The model under review builds one solid part; all positions refer to its coordinate system, in mm. Face numbers are marked on the shaded views. A direction names the side the tool comes from. Round coordinates to 2 decimals unless told otherwise and drop trailing zeros. Loops run counter-clockwise (first coordinate to the right, second up) from the corner with the lowest first, then second, coordinate; pieces in that order, holes last. Notation, with made-up numbers: M -30.75,21.5 L 7.25,21.5 A7 ccw 7.25,27.5 Z; hole C 62,63.5 d5. An arc over 180 degrees is marked long. Use a Markdown table: item, result. Add a question column.
```python
from build123d import *

# Parameters (mm, degrees)
SKETCH1_R                = 5.875
BASE_FLANGE2_DEPTH       = 2.85
TAB1_START               = -2.85
TAB1_DEPTH               = 2.85
FILLET1_R                = 0.5
CIRPATTERN1_COUNT        = 10
FILLET1_OF_CIRPATTERN1_R = 0.5
CUT_EXTRUDE1_DEPTH       = 13.516657182


# Read off the part's stored shape, not the designer's step: Tab1
# Sheet-metal steps are written as plain solids
with BuildPart() as part:
    # Sketch1 → Base-Flange2 (new body)
    with BuildSketch(Plane(origin=(0, 0, 0), x_dir=(1, 0, 0), z_dir=(0, 1, 0))):
        with Locations(Location((0, 0, 0), (0, 0, 270))):
            Circle(SKETCH1_R)
    extrude(amount=-BASE_FLANGE2_DEPTH)

    # Tab1 outline → Tab1 (add)
    with BuildSketch(Plane(origin=(0, 0, 0), x_dir=(1, 0, 0), z_dir=(0, 1, 0)).offset(TAB1_START)):
        with BuildLine():
            ThreePointArc((0.4, 8.79090439), (0, 8.8), (-0.4, 8.79090439))
            ThreePointArc((-0.4, 8.79090439), (-1.1629301, 7.310892011), (-1.5, 5.680283884))
            ThreePointArc((-1.5, 5.680283884), (0, 5.875), (1.5, 5.680283884))
            ThreePointArc((1.5, 5.680283884), (1.1629301, 7.310892011), (0.4, 8.79090439))
        make_face()
    tab1 = extrude(amount=TAB1_DEPTH)

    # Fillet1
    fillet1_edges = [part.edges().sort_by_distance(p)[0] for p in [
        (-1.5, -1.425, -5.680283884),
        (-0.4, -1.425, -8.79090439),
        (0.4, -1.425, -8.79090439),
        (1.5, -1.425, -5.680283884),
    ]]
    fillet(fillet1_edges, radius=FILLET1_R)

    # CirPattern1: Tab1 ×10 about axis
    cirpattern1_axis = Axis((0, 0, 0), (0, 1, 0))
    for i in range(1, CIRPATTERN1_COUNT):
        add(tab1.rotate(cirpattern1_axis, i * 360 / CIRPATTERN1_COUNT))

    # Fillet1 of CirPattern1
    fillet1_of_cirpattern1_edges = [part.edges().sort_by_distance(p)[0] for p in [
        (-4.552312587, -1.425, -3.713768317),
        (-5.490770753, -1.425, -6.876876947),
        (-4.843557157, -1.425, -7.347105148),
        (-2.125261604, -1.425, -5.477124073),
        (-5.865796494, -1.425, -0.328719479),
        (-8.484253702, -1.425, -2.336116246),
        (-8.237040106, -1.425, -3.096961459),
        (-4.938745511, -1.425, -3.181889027),
        (-4.938745511, -1.425, 3.181889027),
        (-8.237040106, -1.425, 3.096961459),
        (-8.484253702, -1.425, 2.336116246),
        (-5.865796494, -1.425, 0.328719479),
        (-2.125261604, -1.425, 5.477124073),
        (-4.843557157, -1.425, 7.347105148),
        (-5.490770753, -1.425, 6.876876947),
        (-4.552312587, -1.425, 3.713768317),
        (1.5, -1.425, 5.680283884),
        (0.4, -1.425, 8.79090439),
        (-0.4, -1.425, 8.79090439),
        (-1.5, -1.425, 5.680283884),
        (4.552312587, -1.425, 3.713768317),
        (5.490770753, -1.425, 6.876876947),
        (4.843557157, -1.425, 7.347105148),
        (2.125261604, -1.425, 5.477124073),
        (5.865796494, -1.425, 0.328719479),
        (8.484253702, -1.425, 2.336116246),
        (8.237040106, -1.425, 3.096961459),
        (4.938745511, -1.425, 3.181889027),
        (4.938745511, -1.425, -3.181889027),
        (8.237040106, -1.425, -3.096961459),
        (8.484253702, -1.425, -2.336116246),
        (5.865796494, -1.425, -0.328719479),
        (2.125261604, -1.425, -5.477124073),
        (4.843557157, -1.425, -7.347105148),
        (5.490770753, -1.425, -6.876876947),
        (4.552312587, -1.425, -3.713768317),
    ]]
    fillet(fillet1_of_cirpattern1_edges, radius=FILLET1_OF_CIRPATTERN1_R)

    # Sketch11 → Cut-Extrude1 (cut, through all)
    with BuildSketch(Plane(origin=(0, 0, 0), x_dir=(1, 0, 0), z_dir=(0, 1, 0))):
        with BuildLine():
            Line((-1.122497216, 0.75), (1.122497216, 0.75))
            ThreePointArc((1.122497216, 0.75), (0, -1.35), (-1.122497216, 0.75))
        make_face()
    extrude(amount=-CUT_EXTRUDE1_DEPTH, mode=Mode.SUBTRACT)


solid = part.part
```
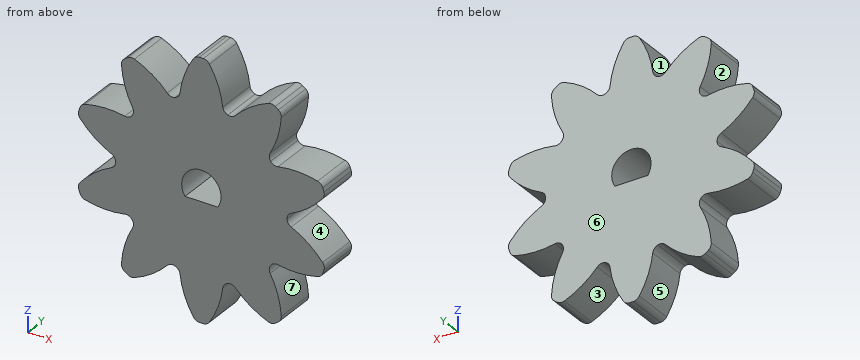
(1) To check wall thickness, follow probe 1 along X at (y, z) = (-1.55, 0) (3 decimals); probe 2 along Z at (x, y) = (0, -1.5); probe 3 along X at (y, z) = (-0.95, 5.75). State the ranges of each line that lie inside material, in increasing order.
(2) Consider section A-A, the plane x = -7. Give the boundary of the cut face in (y, z), then the cut area to 3 significant figures.
(3) For the marked faces 1, 2, 3 and 4, list the 3-axis set-ups (+Z, -Z, +X, -X, +Y, -Y) from which the entire face can be reached by the end or side of a thin tool; tool diameter is ignored.
(4) Consider section C-C, the plane x = 3.25. Give the boundary of the cut face in (y, z), then the cut area to 3 significant figures.
(5) Consider section B-B, the plane z = -5.25. Give the boundary of the cut face in (x, y), then the cut area to 3 significant figures.
(6) Insertion check: pin 1 Ø1.5 at (x, y) = (-2.5, -2) entering from -Z; pin 2 Ø1.5 at (x, y) = (-1.5, -2) entering from +Z; pin 3 Ø1.5 at (x, y) = (4.5, -0.5) entering from -Z. Each pin has a flat end and moves straight along its axis. Give the tip position at first contact, or say it passes through.
(7) Draft analysis for pull direction X (two halves, no side actions). For the marked faces 5, 6 and 7, state which applies: released by +X, released by -X, zero draft, split by the parting line, or undercut.
Found:
| question | item | result |
|---|---|---|
| 1 | probe 1 | x = -5.875 to -1.35, 1.35 to 5.875 |
| 1 | probe 2 | z = -8.8 to -0.75, 1.35 to 8.8 |
| 1 | probe 3 | x = -5.37 to -2.37, -1.58 to 1.58, 2.37 to 5.37 |
| 2 | outline | M -2.85,-3.34 L 0,-3.34 L 0,-0.93 L -2.85,-0.93 Z; M -2.85,0.93 L 0,0.93 L 0,3.34 L -2.85,3.34 Z |
| 2 | area | 13.8 mm^2 |
| 3 | face 1 | +Z, +Y, -Y |
| 3 | face 2 | -X, +Y, -Y |
| 3 | face 3 | -Z, +Y, -Y |
| 3 | face 4 | +X, +Y, -Y |
| 4 | outline | M -2.85,-6.52 L 0,-6.52 L 0,6.52 L -2.85,6.52 Z |
| 4 | area | 37.2 mm^2 |
| 5 | outline | M -5.24,-2.85 L 5.24,-2.85 L 5.24,0 L -5.24,0 Z |
| 5 | area | 29.9 mm^2 |
| 6 | pin 1 | stops at z = -6.52 |
| 6 | pin 2 | stops at z = 8.23 |
| 6 | pin 3 | stops at z = -7.29 |
| 7 | face 5 | undercut |
| 7 | face 6 | zero draft |
| 7 | face 7 | released by +X |
